The listing builds one solid part. Answer for the finished solid, in the listing's coordinates (mm). Face numbers are marked on the shaded views. Coordinates: 2 decimals unless noted, no trailing zeros. Write each loop counter-clockwise with the first axis right and the second up, starting at its lowest first coordinate (ties: lowest second). Pieces come first, ordered by that corner, then holes. Notation, with made-up numbers: M -39.5,71.25 L -21.5,71.25 A30 ccw -21.5,106.25 Z; hole C 47,6 d6. An arc over 180 degrees is marked long. Answer as a JSON object with one key per item and string values. Group by question number.
from build123d import *

# Parameters (mm, degrees)
SKETCH1_W           = 30
SKETCH1_H           = 30
BOSS_EXTRUDE1_DEPTH = 58
SKETCH2_R           = 5.5
SKETCH2_R_2         = 1.25
CUT_EXTRUDE1_DEPTH  = 10
SKETCH3_R           = 5.5
CUT_EXTRUDE2_DEPTH  = 49
SKETCH4_R           = 1.25
CUT_EXTRUDE3_DEPTH  = 8
FILLET1_R           = 5


with BuildPart() as part:
    # Sketch1 → Boss-Extrude1 (new body)
    with BuildSketch(Plane(origin=(0, 0, 0), x_dir=(1, 0, 0), z_dir=(0, 1, 0))):
        Rectangle(SKETCH1_W, SKETCH1_H)
    extrude(amount=BOSS_EXTRUDE1_DEPTH)

    # Sketch2 → Cut-Extrude1 (cut)
    with BuildSketch(Plane(origin=(0, 58, 0), x_dir=(1, 0, 0), z_dir=(0, 1, 0))):
        Circle(SKETCH2_R)
        with Locations((8, 0)):
            Circle(SKETCH2_R_2)
        with Locations((-8, 0)):
            Circle(SKETCH2_R_2)
    extrude(amount=-CUT_EXTRUDE1_DEPTH, mode=Mode.SUBTRACT)

    # Sketch3 → Cut-Extrude2 (cut, through all)
    with BuildSketch(Plane(origin=(0, 48, 0), x_dir=(1, 0, 0), z_dir=(0, 1, 0))):
        Circle(SKETCH3_R)
    extrude(amount=-CUT_EXTRUDE2_DEPTH, mode=Mode.SUBTRACT)

    # Sketch4 → Cut-Extrude3 (cut)
    with BuildSketch(Plane.XY.offset(15)):
        with Locations((0, 47)):
            Circle(SKETCH4_R)
        with Locations((0, 11)):
            Circle(SKETCH4_R)
    cut_extrude3 = extrude(amount=-CUT_EXTRUDE3_DEPTH, mode=Mode.SUBTRACT)

    # Mirror1: Cut-Extrude3 across plane
    add(cut_extrude3.mirror(Plane.XY), mode=Mode.SUBTRACT)

    # Fillet1
    fillet1_edges = [part.edges().sort_by_distance(p)[0] for p in [
        (15, 29, 15),
        (-15, 29, 15),
        (-15, 29, -15),
        (15, 29, -15),
    ]]
    fillet(fillet1_edges, radius=FILLET1_R)


solid = part.part
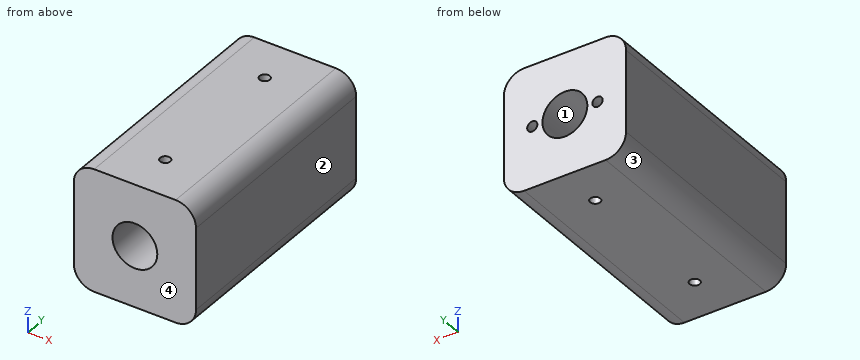
Item 1: A cutting plane is placed at D-D, the plane x = 3.5. Write down the section's boundary in (y, z), and give its area (3 significant figures).
Item 2: For a pull along X with two mould halves and no side action, classify the marked faces 1, 2, 3 and 4 as +X half, -X half, draft (parallel to the pull), parting line (faces both ways), or undercut.
Item 3: A cutting plane is placed at A-A, the plane x = 0. Write down the section's boundary in (y, z), and give its area (3 significant figures).
Item 4: A cutting plane is placed at B-B, the plane y = 47. Write down the section's boundary in (x, z), and give its area (3 significant figures).
Item 5: Consider L1, parallel to Y at x = 0, z = -10.5; L2, parallel to X at y = 25, z = -1; L3, parallel to Z at x = -4.25, y = 26. Determine where each line is inside the solid, lowest interval first. Write a range as from..to.
Item 6: Flat-ended cylindrical pins translate along their axes: pin 1 Ø0.8 at (x, y) = (-0.5, 10.5) entering from +Z; pin 2 Ø1.2 at (x, z) = (8, 0) entering from +Y; pin 3 Ø2 at (x, y) = (0, 47) entering from -Z. Find the tip coordinate at first contact, or state that the pin passes through.
Item 7: A cutting plane is placed at C-C, the plane z = -2.75. Write down the section's boundary in (x, y), and give its area (3 significant figures).
Answer:
{
 "1": {"outline": "M 0,-15 L 58,-15 L 58,-4.24 L 0,-4.24 Z; M 0,4.24 L 58,4.24 L 58,15 L 0,15 Z", "area": "1,250 mm2"},
 "2": {"face 1": "undercut", "face 2": "+X half", "face 3": "-X half", "face 4": "draft"},
 "3": {"outline": "M 0,-15 L 9.75,-15 L 9.75,-7 L 12.25,-7 L 12.25,-15 L 45.75,-15 L 45.75,-7 L 48.25,-7 L 48.25,-15 L 58,-15 L 58,-5.5 L 0,-5.5 Z; M 0,5.5 L 58,5.5 L 58,15 L 48.25,15 L 48.25,7 L 45.75,7 L 45.75,15 L 12.25,15 L 12.25,7 L 9.75,7 L 9.75,15 L 0,15 Z", "area": "1,020 mm2"},
 "4": {"outline": "M -15,-10 A5 ccw -10,-15 L -1.25,-15 L -1.25,-7 L 1.25,-7 L 1.25,-15 L 10,-15 A5 ccw 15,-10 L 15,10 A5 ccw 10,15 L 1.25,15 L 1.25,7 L -1.25,7 L -1.25,15 L -10,15 A5 ccw -15,10 Z; hole C 0,0 d11", "area": "744 mm2"},
 "5": {"L1": "0..9.75, 12.25..45.75, 48.25..58", "L2": "-15..-5.41, 5.41..15", "L3": "-15..-3.49, 3.49..15"},
 "6": {"pin 1": "z = 7", "pin 2": "y = 48", "pin 3": "z = -7"},
 "7": {"outline": "M -15,0 L -4.76,0 L -4.76,58 L -15,58 Z; M 4.76,0 L 15,0 L 15,58 L 4.76,58 Z", "area": "1,190 mm2"}
}
